Job drawing, mm, ordinate dimensions from the low corner. One solid piece. A direction names the side the tool comes from. Coordinates: 2 decimals unless noted, no trailing zeros. Order: outer loops, then holes, each group sorted by start corner. A loop starts at its lowest first (then second) coordinate and runs counter-clockwise, first axis right, second up. Notation, with made-up numbers: (-18, 57) - (32, 57) arc R15 cw to (32, 80) - close; hole circle Ø2 at (76, 22). An arc over 180 degrees is marked (long way). Return JSON: item names as keys, results as strings.
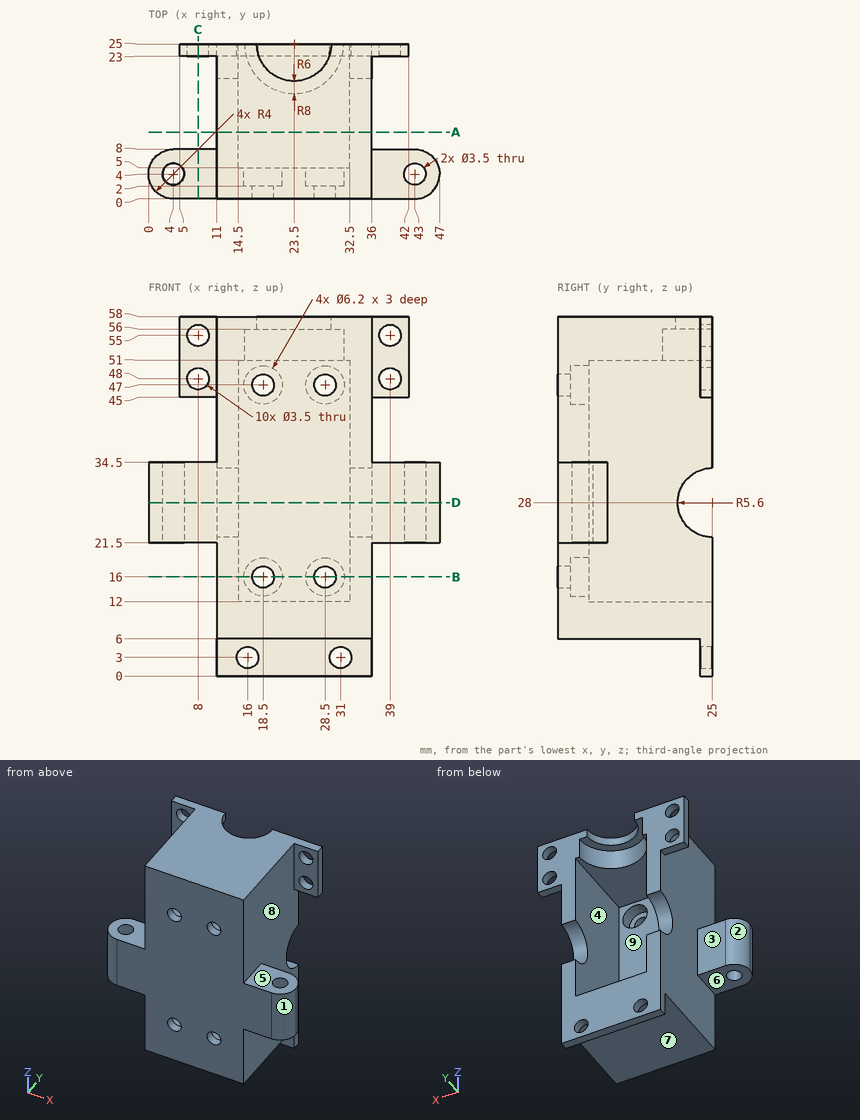
1. Cut at D-D on z = 28. State how many separate pieces and enclosed holes the cut face has, plus the area to 3 significant figures.
Check values:
{"separate pieces": "1", "enclosed holes": "2", "area": "369 mm²"}
2. Cut at C-C on x = 8. Give the cut face in (y, z).
Check values:
{"outline": "(0, 21.5) - (8, 21.5) - (8, 34.5) - (0, 34.5) - close; (23, 45) - (25, 45) - (25, 46.25) - (23, 46.25) - close; (23, 49.75) - (25, 49.75) - (25, 53.25) - (23, 53.25) - close; (23, 56.75) - (25, 56.75) - (25, 58) - (23, 58) - close"}
3. Cut at B-B on z = 16. Give the cut face in (x, y).
Check values:
{"outline": "(11, 0) - (16.75, 0) - (16.75, 2) - (15.4, 2) - (15.4, 5) - (14.5, 5) - (14.5, 25) - (11, 25) - close; (20.25, 0) - (26.75, 0) - (26.75, 2) - (25.4, 2) - (25.4, 5) - (21.6, 5) - (21.6, 2) - (20.25, 2) - close; (30.25, 0) - (36, 0) - (36, 25) - (32.5, 25) - (32.5, 5) - (31.6, 5) - (31.6, 2) - (30.25, 2) - close"}
4. Mould opens along X. For the marked faces 1, 2, 3 and 4 say: pulls with the +X half, pulls with the -X half, needs draft (parallel to the pull), parting line crosses it, or undercut.
Check values:
{"face 1": "pulls with the +X half", "face 2": "pulls with the -X half", "face 3": "needs draft", "face 4": "undercut"}
5. Cut at A-A on y = 10.75. Give the cut face in (x, z), plus the area to 3 significant figures.
Check values:
{"outline": "(11, 6) - (36, 6) - (36, 58) - (11, 58) - close; hole (14.5, 12) - (32.5, 12) - (32.5, 51) - (14.5, 51) - close", "area": "598 mm²"}
6. Probe L1, parallel to X at y = 3.4, z = 16; L2, parallel to X at y = 0.7, z = 16; L3, parallel to X at y = 21.75, z = 41.5. List the from-to ranges inside material, lowest first.
Check values:
{"L1": "11 to 15.4, 21.6 to 25.4, 31.6 to 36", "L2": "11 to 16.75, 20.25 to 26.75, 30.25 to 36", "L3": "11 to 14.5, 32.5 to 36"}
7. Drop flat-ended pins along their axis: pin 1 (6 mm diameter, centred on x = 36.5, y = 20, fed in from -Z); pin 2 (5 mm diameter, centred on x = 29.5, z = 15, fed in from +Y); pin 3 (2.5 mm diameter, centred on x = 7, y = 2, fed in from +Z). Give the stop position or say it passes through.
Check values:
{"pin 1": "z = 6", "pin 2": "y = 5", "pin 3": "z = 34.5"}
8. Tool access for the marked faces 5, 6, 7, 8 and 9: list every direction of +Z, -Z, +X, -X, +Y, -Y with a clear straight run to the whole face (end or side of a thin tool).
Check values:
{"face 5": "+Z, +X, +Y, -Y", "face 6": "-Z, -X, +Y, -Y", "face 7": "-Z, +X, -X, -Y", "face 8": "+X", "face 9": "+Y"}
